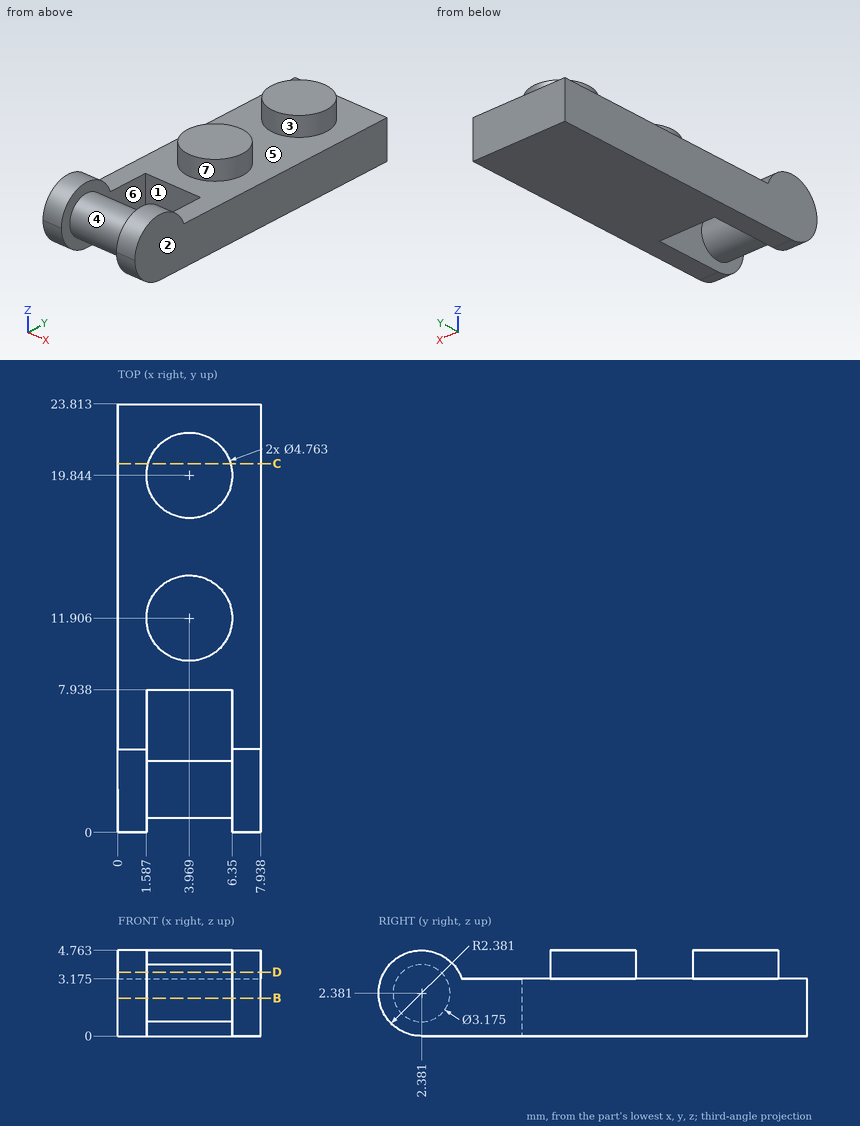
Here's the drawing with two shaded views (mm, measured from the low corner). I have some questions. A direction names the side the tool comes from. Coordinates: 2 decimals unless noted, no trailing zeros. Order: outer loops, then holes, each group sorted by start corner. A loop starts at its lowest first (then second) coordinate and runs counter-clockwise, first axis right, second up. Notation, with made-up numbers: (-20.5, 52.25) -> (-11.5, 52.25) arc R14 ccw to (-11.5, 74.25) -> close; hole circle Ø7 at (-37.5, 60). An arc over 180 degrees is marked (long way). Write each question's results on one line, items separated by ' | '.
Item 1: Which directions (+Z, -Z, +X, -X, +Y, -Y) give clear straight access to the entire face, cutting with the end or side of a thin tool? Please do the marked faces 1, 2 and 3.
Results are:
face 1: +Z, -Z | face 2: +Z, -Z, +X, +Y, -Y | face 3: +Z
Item 2: I'm going to push flat-ended pins straight in: pin 1 Ø3 at (x, y) = (6.5, 4) entering from +Z; pin 2 Ø2 at (x, z) = (5, 2.5) entering from -Y. Where does each tip first touch, or does it pass through?
Results are:
pin 1: z = 4.76 | pin 2: y = 0.79
Item 3: If we mould it in two halves opening along X, with no side actions, what happens to the marked faces 4, 5, 6 and 7? For each: +X half, -X half, draft (parallel to the pull), parting line (faces both ways), or undercut.
Results are:
face 4: undercut | face 5: draft | face 6: undercut | face 7: parting line
Item 4: I want a section at C-C, the plane y = 20.5. Write out the boundary of the cut face in (x, z) (1 decimal).
Results are:
outline: (0, 0) -> (7.9, 0) -> (7.9, 3.2) -> (6.3, 3.2) -> (6.3, 4.8) -> (1.7, 4.8) -> (1.7, 3.2) -> (0, 3.2) -> close
Item 5: I want a section at B-B, the plane z = 2.1. Write out the boundary of the cut face in (x, y).
Results are:
outline: (0, 0.02) -> (1.59, 0.02) -> (1.59, 0.82) -> (6.35, 0.82) -> (6.35, 0.02) -> (7.94, 0.02) -> (7.94, 23.81) -> (0, 23.81) -> close; hole (1.59, 3.94) -> (6.35, 3.94) -> (6.35, 7.94) -> (1.59, 7.94) -> close
Item 6: If I drill on line 1 along X through (y, z) = (1.5, 0.35); line 2 along Y through (x, z) = (6, 2.5) (1 decimal); line 3 along Y through (x, z) = (5.25, 0.3), over which ranges is the centre line in solid material (lowest first)?
Results are:
line 1: 0 to 1.59, 6.35 to 7.94 | line 2: 0.8 to 4, 7.9 to 23.8 | line 3: 7.94 to 23.81
Item 7: I want a section at D-D, the plane z = 3.55. Count the separate pieces of the cut face and the enclosed holes in it.
Results are:
separate pieces: 3 | enclosed holes: 0
